Build history of the part. All positions in model axes, mm. A direction names the side the tool comes from. Round coordinates to 2 decimals unless told otherwise and drop trailing zeros. Write each loop counter-clockwise with the first axis right and the second up, starting at its lowest first coordinate (ties: lowest second). Pieces come first, ordered by that corner, then holes. Notation, with made-up numbers: (39.25, 4) -> (82.25, 4) arc R29 cw to (82.25, 26) -> close; hole circle Ø7 at (70.5, 85.5). An arc over 180 degrees is marked (long way). Answer in a Markdown table with one row per item.
```python
from build123d import *

# Parameters (mm, degrees)
CHAMFER1_SIZE = 0.3


with BuildPart() as part:
    # Sketch1 → Revolve1 (revolve)
    with BuildSketch(Plane(origin=(0, 0, 0), x_dir=(1, 0, 0), z_dir=(0, 1, 0))):
        Polygon((-7.987, 0.5), (-7.987, 5.115), (-9.77, 5.115), (-12.188305192, 2.696694808), (-9.77, 0.278389617), (-9.375, 0.278389617), (-9.375, -0.278389617), (-9.77, -0.278389617), (-12.188305192, -2.696694808), (-9.77, -5.115), (-7.987, -5.115), (-7.987, -0.5), (-6.945, -0.5), (-6.945, 0.5), align=None)
    revolve(axis=Axis((0, 0, -5.115), (0, 0, 1)))

    # Chamfer1
    chamfer1_edges = [part.edges().sort_by_distance(p)[0] for p in [
        (7.987, 0, 5.115),
        (7.987, 0, -5.115),
    ]]
    chamfer(chamfer1_edges, length=CHAMFER1_SIZE)


solid = part.part
```
Q1. Drop flat-ended pins along their axis: P1, Ø6, axis at y = 3, z = -3.5, coming from the -X side; P2, Ø1, axis at x = -2.5, z = -3.5, coming from the +Y side. Give the stop position or say it passes through.
A:
| item | result |
|---|---|
| P1 | x = -12.19 |
| P2 | y = 11.63 |
Q2. Two-plate mould, pull along Y, no slides. Class faces 4 (the conical face through (2.15, 9.69, -4.96)), 5 (the flat face through (4.4, 7.2, 5.115)), 6 (the cylindrical face through (5.887, -5.398, -2.688)): released by +Y, released by -Y, zero draft, split by the parting line, or undercut.
A:
| item | result |
|---|---|
| face 4 | split by the parting line |
| face 5 | zero draft |
| face 6 | undercut |
Q3. Wall check: line 1 (Y direction, x = 0, z = -0.05) (3 decimals); line 2 (Y direction, x = 6.25, z = 3). Give the ranges that are in metal, low to high. Write a range as [from, to].
A:
| item | result |
|---|---|
| line 1 | [-9.375, -6.945], [6.945, 9.375] |
| line 2 | [-10.11, -4.97], [4.97, 10.11] |
Q4. Saw through at C-C on z = 1.25. Write the cut outline in (x, y), plus the area to 3 significant figures.
A:
| item | result |
|---|---|
| outline | circle Ø21.48 at (0, 0); hole circle Ø15.97 at (0, 0) |
| area | 162 mm² |
Q5. Saw through at D-D on z = 3.25. Write the cut outline in (x, y) (3 decimals).
A:
| item | result |
|---|---|
| outline | circle Ø23.27 at (0, 0); hole circle Ø15.974 at (0, 0) |
Q6. Which spindle directions (+Z, -Z, +X, -X, +Y, -Y) get a long thin tool onto all of the face, cutting with end or side? Do faces 1 (the flat face through (-2, -7, -0.5)), 2 (the flat face through (2, -7, 0.5)), 3 (the conical face through (2.151, 9.685, 0.43)). Say none if no direction does.
A:
| item | result |
|---|---|
| face 1 | -Z |
| face 2 | +Z |
| face 3 | none |
